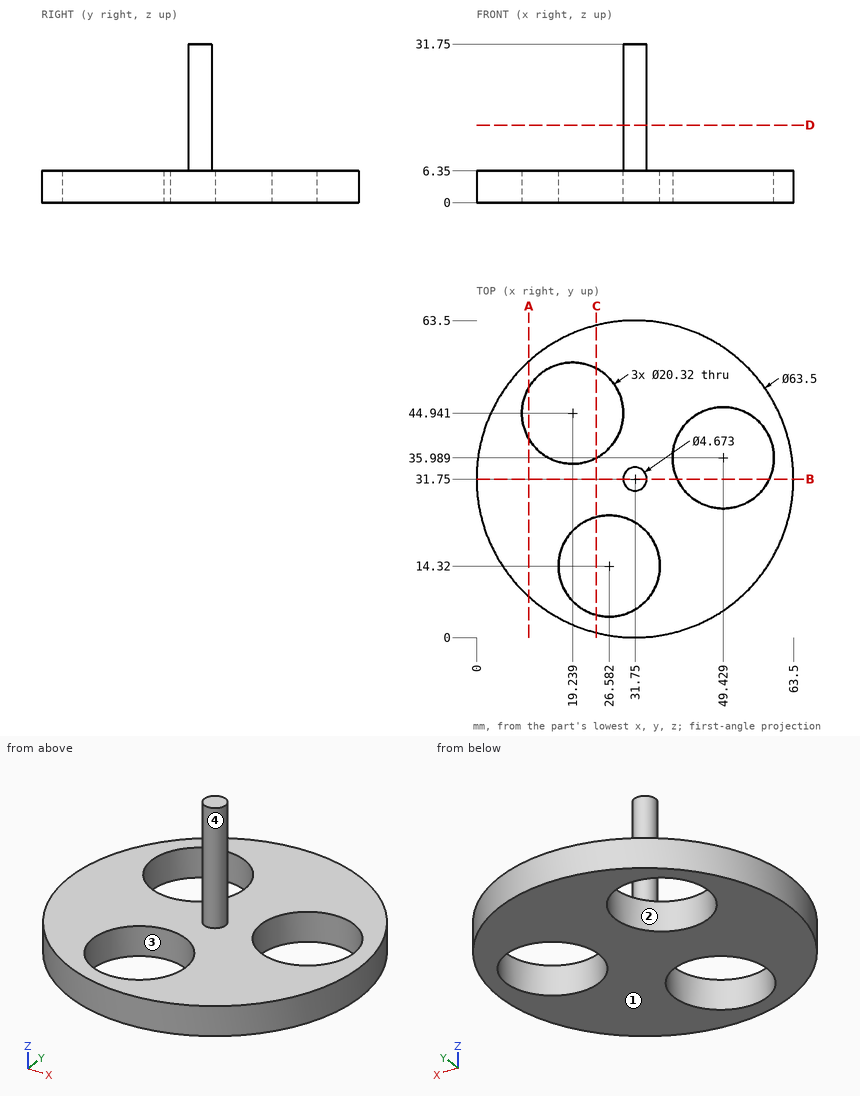
The drawing under review shows one solid part. Ordinate dimensions are in mm from its lowest x, y, z. Coordinates: 2 decimals unless noted, no trailing zeros. Loops run counter-clockwise (first coordinate to the right, second up) from the corner with the lowest first, then second, coordinate; pieces in that order, holes last.
Item 1: Clearance check with flat-ended pins moving along their axes: pin 1 (23.5 mm diameter, centred on x = 49.43, y = 35.99, fed in from +Z); pin 2 (12 mm diameter, centred on y = 29.5, z = 18, fed in from -X); pin 3 (3 mm diameter, centred on x = 52, z = 7.5, fed in from +Y). State where each tip first meets the part, or that it passes through.
Completed:
pin 1: stops at z = 6.35
pin 2: stops at x = 29.41
pin 3: stops at y = 56.97
Item 2: Add section C-C (x = 24). Give the number of separate pieces and of enclosed holes in the cut face, and give its area (3 significant figures).
Completed:
separate pieces: 3
enclosed holes: 0
area: 152 mm2
Item 3: Add section B-B (y = 31.75). Write out the cut boundary in (x, z), and give its area (3 significant figures).
Completed:
outline: (0, 0) - (40.2, 0) - (40.2, 6.35) - (34.09, 6.35) - (34.09, 31.75) - (29.41, 31.75) - (29.41, 6.35) - (0, 6.35) - close; (58.66, 0) - (63.5, 0) - (63.5, 6.35) - (58.66, 6.35) - close
area: 405 mm2
Item 4: Add section A-A (x = 10.5). Write out the cut boundary in (y, z), and give its area (3 significant figures).
Completed:
outline: (8.16, 0) - (39.76, 0) - (39.76, 6.35) - (8.16, 6.35) - close; (50.12, 0) - (55.34, 0) - (55.34, 6.35) - (50.12, 6.35) - close
area: 234 mm2
Item 5: Add section D-D (z = 15.5). Write out the cut boundary in (x, y).
Completed:
outline: circle Ø4.67 at (31.75, 31.75)
Item 6: Wall thickness on L1, parallel to Z at x = 34, y = 28; L2, parallel to X at y = 7, z = 3 (1 decimal); L3, parallel to X at y = 21, z = 2 (1 decimal): over which ranges is each line inside the solid? List them lowest first.
Completed:
L1: z = 0 to 6.35
L2: x = 11.9 to 19.5, 33.6 to 51.6
L3: x = 1.9 to 18.9, 34.2 to 61.6
Item 7: Draft analysis for pull direction Y (two halves, no side actions). For the marked faces 1, 2, 3 and 4, state which applies: pulls with the +Y half, pulls with the -Y half, needs draft (parallel to the pull), parting line crosses it, or undercut.
Completed:
face 1: needs draft
face 2: undercut
face 3: undercut
face 4: parting line crosses it
